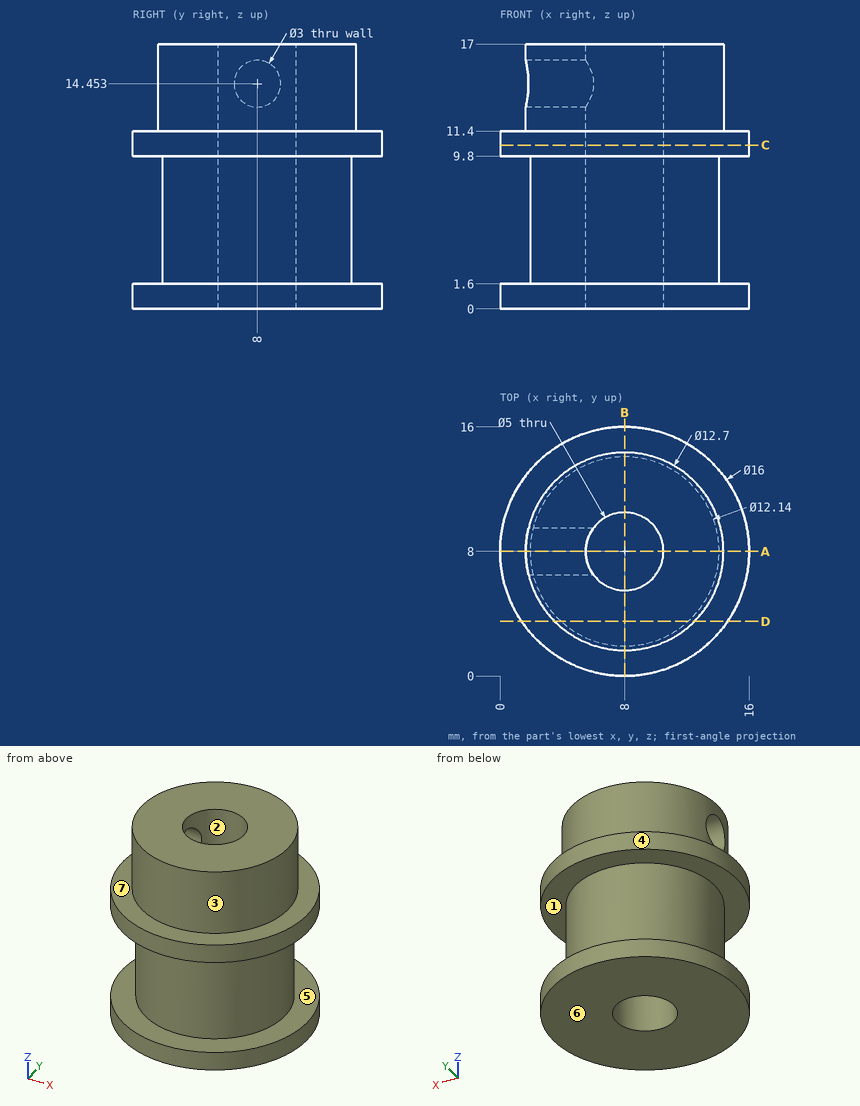
Here's the drawing with two shaded views (mm, measured from the low corner). I have some questions. A direction names the side the tool comes from. Round coordinates to 2 decimals unless told otherwise and drop trailing zeros. Loops run counter-clockwise (first coordinate to the right, second up) from the corner with the lowest first, then second, coordinate; pieces in that order, holes last.
1. Will these pins go through, and if not, where does the flat tip stop? pin 1 (8 mm diameter, centred on x = 8, y = 8, fed in from +Z); pin 2 (5 mm diameter, centred on y = 6, z = 4, fed in from +X); pin 3 (1 mm diameter, centred on y = 4.5, z = 14, fed in from -X); pin 4 (1.8 mm diameter, centred on y = 8, z = 14.45, fed in from -X).
Answers:
pin 1: stops at z = 17
pin 2: stops at x = 15.89
pin 3: stops at x = 2.4
pin 4: stops at x = 10.33
2. Suppose I cut it at C-C, the plane z = 10.5. Please give me the cut outline in (x, y), and give its area (3 significant figures).
Answers:
outline: circle Ø16 at (8, 8); hole circle Ø5 at (8, 8)
area: 181 mm2
3. Thinking about a two-plate mould opening in Z: for the marked faces 4, 5, 6 and 7, which applies, released by +Z, released by -Z, zero draft, split by the parting line, or undercut?
Answers:
face 4: zero draft
face 5: undercut
face 6: released by -Z
face 7: released by +Z
4. Suppose I cut it at B-B, the plane x = 8. Please give me the cut outline in (y, z).
Answers:
outline: (0, 0) - (5.5, 0) - (5.5, 17) - (1.65, 17) - (1.65, 11.4) - (0, 11.4) - (0, 9.8) - (1.93, 9.8) - (1.93, 1.6) - (0, 1.6) - close; (10.5, 0) - (16, 0) - (16, 1.6) - (14.07, 1.6) - (14.07, 9.8) - (16, 9.8) - (16, 11.4) - (14.35, 11.4) - (14.35, 17) - (10.5, 17) - close
5. If I drill on probe 1 along X at (y, z) = (8, 12); probe 2 along Z at (x, y) = (14.5, 4.5); probe 3 along Y at (x, z) = (8, 3.75), over which ranges is the centre line in solid material (lowest first)?
Answers:
probe 1: x = 1.65 to 5.5, 10.5 to 14.35
probe 2: z = 0 to 1.6, 9.8 to 11.4
probe 3: y = 1.93 to 5.5, 10.5 to 14.07
6. Suppose I cut it at D-D, the plane y = 3.5. Please give me the cut outline in (x, z), and give its area (3 significant figures).
Answers:
outline: (1.39, 0) - (14.61, 0) - (14.61, 1.6) - (12.07, 1.6) - (12.07, 9.8) - (14.61, 9.8) - (14.61, 11.4) - (12.48, 11.4) - (12.48, 17) - (3.52, 17) - (3.52, 11.4) - (1.39, 11.4) - (1.39, 9.8) - (3.93, 9.8) - (3.93, 1.6) - (1.39, 1.6) - close
area: 159 mm2
7. Suppose I cut it at A-A, the plane y = 8. Please give me the cut outline in (x, z), and give its area (3 significant figures).
Answers:
outline: (0, 0) - (5.5, 0) - (5.5, 12.95) - (1.65, 12.95) - (1.65, 11.4) - (0, 11.4) - (0, 9.8) - (1.93, 9.8) - (1.93, 1.6) - (0, 1.6) - close; (1.65, 15.95) - (5.5, 15.95) - (5.5, 17) - (1.65, 17) - close; (10.5, 0) - (16, 0) - (16, 1.6) - (14.07, 1.6) - (14.07, 9.8) - (16, 9.8) - (16, 11.4) - (14.35, 11.4) - (14.35, 17) - (10.5, 17) - close
area: 125 mm2
8. For the marked faces 1, 2 and 3, which set-ups out of +Z, -Z, +X, -X, +Y, -Y let a thin tool reach every point of the face, with its end or its side?
Answers:
face 1: none
face 2: +Z, -Z
face 3: +Z
